```python
from build123d import *

# Parameters (mm, degrees)
F0_W      = 5
F0_H      = 10
F1_DEPTH  = 2
F2_R      = 0.25
F4_DEPTH  = 2.45
F5_W      = 0.8
F5_H      = 4.5
F6_DEPTH  = 2.45
F7_W      = 2
F7_H      = 3.1
F8_DEPTH  = 0.8
F9_W      = 1.45
F9_H      = 1
F10_DEPTH = 0.8


# Not quite as in the source:
# - a feature names something its author has since deleted; it is built from what else it names


with BuildPart() as f1:
    # F0 (on Top) → F1 (new body)
    with BuildSketch(Plane.XY):
        Rectangle(F0_W, F0_H)
    extrude(amount=F1_DEPTH)

    # F2
    f2_edges = [f1.edges().sort_by_distance(p)[0] for p in [
        (2.5, 5, 1),
        (-2.5, -5, 1),
        (0, 5, 0),
        (2.5, 0, 0),
        (-2.5, 0, 0),
        (0, -5, 0),
        (-2.5, 5, 1),
        (2.5, -5, 1),
    ]]
    fillet(f2_edges, radius=F2_R)

    # F3 (on Front) → F4 (join, symmetric)
    with BuildSketch(Plane.XZ):
        Polygon((0.8, 4.4), (0.8, 2), (1.4, 2), (1.4, 3.4), (2.2, 3.4), (1.4, 4.4), align=None)
    extrude(amount=F4_DEPTH, both=True)

    # F5 (on Front) → F6 (join, symmetric)
    with BuildSketch(Plane.XZ):
        with Locations((-1, 4.25)):
            Rectangle(F5_W, F5_H)
    extrude(amount=F6_DEPTH, both=True)

    # F7 (on face) → F8 (cut, through all)
    with BuildSketch(Plane(origin=(-1.4, 0, 0), x_dir=(0, -1, 0), z_dir=(-1, 0, 0))):
        with Locations((0, 4.95)):
            Rectangle(F7_W, F7_H)
    extrude(amount=-F8_DEPTH, mode=Mode.SUBTRACT)

    # F9 (on face) → F10 (join)
    with BuildSketch(Plane(origin=(-1.4, 0, 0), x_dir=(0, -1, 0), z_dir=(-1, 0, 0))):
        with Locations((-1.725, 3.9)):
            Rectangle(F9_W, F9_H)
        with Locations((1.725, 3.9)):
            Rectangle(F9_W, F9_H)
    extrude(amount=F10_DEPTH)


solid = f1.part
```
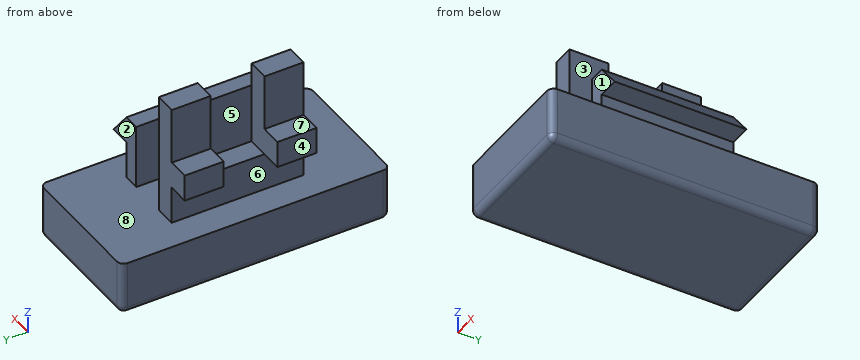
Geometry check sheet. Reference: the model listing, model coordinates, mm. Face numbers are marked on the shaded views. A direction names the side the tool comes from. Coordinates: 2 decimals unless noted, no trailing zeros. Order: outer loops, then holes, each group sorted by start corner. A loop starts at its lowest first (then second) coordinate and runs counter-clockwise, first axis right, second up.
Q1. Sectioned sample at D-D on x = -1.15. Record the cut outline in (y, z), and give its area (3 significant figures).
Reply:
outline: (-5, 0.25) arc R0.25 ccw to (-4.75, 0) - (4.75, 0) arc R0.25 ccw to (5, 0.25) - (5, 2) - (2.45, 2) - (2.45, 6.5) - (1, 6.5) - (1, 3.4) - (-1, 3.4) - (-1, 6.5) - (-2.45, 6.5) - (-2.45, 2) - (-5, 2) - close
area: 35.8 mm2
Q2. Depth check by flat-ended pin: pin 1 Ø2 at (x, y) = (1, -2) entering from +Z; pin 2 Ø1.1 at (y, z) = (-2, 4) entering from -X; pin 3 Ø1.5 at (x, z) = (0, 4.5) entering from -Y. Enter the tip coordinate at first touch or a pass-through.
Reply:
pin 1: stops at z = 4.4
pin 2: stops at x = -2.2
pin 3: stops at y = -2.45
Q3. Thickness scan on probe 1 along X at (y, z) = (-2.25, 3.25); probe 2 along Y at (x, z) = (-1.85, 3.5); probe 3 along Z at (x, y) = (-1.75, -3.5). Record the ranges inside material, lowest first.
Reply:
probe 1: x = -1.4 to -0.6, 0.8 to 1.4
probe 2: y = -2.45 to -1, 1 to 2.45
probe 3: z = 0 to 2
Q4. Sectioned sample at A-A on z = 4. Record the cut outline in (x, y), and give its area (3 significant figures).
Reply:
outline: (-2.2, -2.45) - (-0.6, -2.45) - (-0.6, -1) - (-2.2, -1) - close; (-2.2, 1) - (-0.6, 1) - (-0.6, 2.45) - (-2.2, 2.45) - close; (0.8, -2.45) - (1.72, -2.45) - (1.72, 2.45) - (0.8, 2.45) - close
area: 9.15 mm2
Q5. Sectioned sample at C-C on x = -1.95. Record the cut outline in (y, z).
Reply:
outline: (-5, 0.25) arc R0.25 ccw to (-4.75, 0) - (4.75, 0) arc R0.25 ccw to (5, 0.25) - (5, 2) - (-5, 2) - close; (-2.45, 3.4) - (-1, 3.4) - (-1, 4.4) - (-2.45, 4.4) - close; (1, 3.4) - (2.45, 3.4) - (2.45, 4.4) - (1, 4.4) - close
Q6. Tool access check on the marked faces 1, 2, 3 and 4. Record the directions out of +Z, -Z, +X, -X, +Y, -Y that give a thin tool (end or side, any length) a straight path to the whole face; none if there is none.
Reply:
face 1: +Z, +X, -X, -Y
face 2: +Z, +X, -X, +Y
face 3: +Z, +Y, -Y
face 4: +Z, -X, +Y, -Y
Q7. Draft check along Z on the marked faces 5, 6, 7 and 8. Enter one of: released by +Z, released by -Z, zero draft, split by the parting line, or undercut.
Reply:
face 5: zero draft
face 6: undercut
face 7: released by +Z
face 8: undercut
Q8. Sectioned sample at B-B on z = 2.5. Record the cut outline in (x, y).
Reply:
outline: (-1.4, -2.45) - (-0.6, -2.45) - (-0.6, 2.45) - (-1.4, 2.45) - close; (0.8, -2.45) - (1.4, -2.45) - (1.4, 2.45) - (0.8, 2.45) - close
